Geometry check sheet. Reference: the model listing, model coordinates, mm. A direction names the side the tool comes from. Round coordinates to 2 decimals unless told otherwise and drop trailing zeros. Write each loop counter-clockwise with the first axis right and the second up, starting at its lowest first coordinate (ties: lowest second). Pieces come first, ordered by that corner, then holes. Notation, with made-up numbers: (52.25, -32.5) - (93.25, -32.5) arc R12 cw to (93.25, -24.5) - close; hole circle Ø8 at (-9.5, 66). An arc over 180 degrees is marked (long way). One line per question, with ' | ' between items. Start each with the question number.
from build123d import *

# Parameters (mm, degrees)
F0_R     = 101.314415
F1_DEPTH = 355.6
F2_W     = 103.034616
F2_H     = 254.342378
F3_DEPTH = 318.465123
F4_DEPTH = 381
F5_R     = 12.7


with BuildPart() as f1:
    # F0 (on Top) → F1 (new body)
    with BuildSketch(Plane.XY):
        Circle(F0_R)
    extrude(amount=F1_DEPTH)

    # F2 (on Front) → F3 (join)
    with BuildSketch(Plane.XZ):
        with Locations((0, 162.727058)):
            Rectangle(F2_W, F2_H)
    extrude(amount=-F3_DEPTH)

    # F2 (on Front) → F4 (join)
    with BuildSketch(Plane.XZ):
        with Locations((0, 162.727058)):
            Rectangle(F2_W, F2_H)
    extrude(amount=F4_DEPTH)

    # F5
    f5_edges = [f1.edges().sort_by_distance(p)[0] for p in [
        (-101.314415, 0, 0),
        (51.517308, -234.119313, 35.555869),
        (51.517308, -234.119313, 289.898247),
        (51.517308, -381, 162.727058),
        (-51.517308, -234.119313, 35.555869),
        (-51.517308, -234.119313, 289.898247),
        (0, -381, 289.898247),
        (-51.517308, -381, 162.727058),
        (0, -381, 35.555869),
    ]]
    fillet(f5_edges, radius=F5_R)


solid = f1.part
Q1. Go/stop test with flat-tipped pins: P1, Ø2, axis at x = 18, y = -123.5, coming from the +Z side; P2, Ø3, axis at y = -301.5, z = 201, coming from the -X side; P3, Ø4, axis at y = 97, z = 58.5, coming from the +X side. Record where each tip stops, or that it passes through.
Q2. Section check D-D, the plane z = 315. Record the cut outline in (x, y), then the cut area to 3 significant figures.
Q3. Section check C-C, the plane y = -182.5. Record the cut outline in (x, z).
Q4. Section check A-A, the plane z = 70.5. Record the cut outline in (x, y), then the cut area to 3 significant figures.
Q5. Thickness scan on line 1 (Z direction, x = -30.5, y = 97); line 2 (X direction, y = -299, z = 163.5); line 3 (Y direction, x = 3, z = 294). Record the ranges inside material, lowest first.
Q6. Section check B-B, the plane x = 0. Record the cut outline in (y, z).
Q7. Set-up check for faces 1 (the cylindrical face through (-47.896, -229.737, 39.375)), 2 (the flat face through (-51.517, -226, 161)), 3 (the flat face through (-51.517, 201, 161)), 4 (the flat face through (51.517, 201, 161)): record each of +Z, -Z, +X, -X, +Y, -Y from which the full face is reachable in a straight line by a thin tool's end or side.
Result sheet:
1) P1: z = 289.9 | P2: x = -51.52 | P3: x = 51.52
2) outline: circle Ø202.63 at (0, 0) | area: 32,200 mm²
3) outline: (-51.52, 48.26) arc R12.7 ccw to (-38.82, 35.56) - (38.82, 35.56) arc R12.7 ccw to (51.52, 48.26) - (51.52, 277.2) arc R12.7 ccw to (38.82, 289.9) - (-38.82, 289.9) arc R12.7 ccw to (-51.52, 277.2) - close
4) outline: (-51.52, -368.3) arc R12.7 ccw to (-38.82, -381) - (38.82, -381) arc R12.7 ccw to (51.52, -368.3) - (51.52, -87.24) arc R101.31 ccw to (51.52, 87.24) - (51.52, 318.47) - (-51.52, 318.47) - (-51.52, 87.24) arc R101.31 ccw to (-51.52, -87.24) - close | area: 84,300 mm²
5) line 1: 35.56 to 289.9 | line 2: -51.52 to 51.52 | line 3: -101.27 to 101.27
6) outline: (-381, 48.26) arc R12.7 ccw to (-368.3, 35.56) - (-101.31, 35.56) - (-101.31, 12.7) arc R12.7 ccw to (-88.61, 0) - (88.61, 0) arc R12.7 ccw to (101.31, 12.7) - (101.31, 35.56) - (318.47, 35.56) - (318.47, 289.9) - (101.31, 289.9) - (101.31, 355.6) - (-101.31, 355.6) - (-101.31, 289.9) - (-368.3, 289.9) arc R12.7 ccw to (-381, 277.2) - close
7) face 1: -Z, -X, -Y | face 2: +Z, -Z, -X, -Y | face 3: +Z, -Z, -X, +Y | face 4: +Z, -Z, +X, +Y
